Source: three-view drawing plus pictorial views. Frame: mm from the lowest corner of the part. A direction names the side the tool comes from. Give positions to 0.01 mm unless a question says otherwise; leave off trailing zeros. Order: outer loops, then holes, each group sorted by start corner. A loop starts at its lowest first (then second) coordinate and runs counter-clockwise, first axis right, second up. Notation, with made-up numbers: M 46,5 L 81,5 A18 cw 81,19 Z; hole C 11,76 d5. An arc over 180 degrees is marked long. Use CSV: the item, a comma, the result in double quotes. Start each with the question number.
1. Pin query (flat end, axial travel): P1, Ø5, axis at y = 7, z = 62, coming from the -X side (1 decimal); P2, Ø4, axis at x = 26.5, z = 35.5, coming from the -Y side; P3, Ø2.5, axis at x = 35, z = 20, coming from the +Y side; P4, Ø8, axis at x = 27.5, z = 44, coming from the +Y side. Return the tip coordinate at first contact, or that it passes through.
2. Mould query, pull axis Z, two halves, no side actions, for the marked faces 4, 5, 6 and 7. Classes: released by +Z, released by -Z, zero draft, split by the parting line, or undercut.
3. Section query D-D, the plane z = 50. Return the cut outline in (x, y).
4. Reachability of the marked faces 1, 2 and 3 from +Z, -Z, +X, -X, +Y, -Y: full face, straight path, thin tool, end or side. Return the list, or none.
5. Line query: line 1 along Z through (x, y) = (14.5, 9.5); line 2 along Y through (x, z) = (46.5, 21.5); line 3 along Z through (x, y) = (23.5, 7.75) (1 decimal). Output: solid intervals per line, ascending. Write a range as [from, to].
6. Section query A-A, the plane x = 35. Return the cut outline in (y, z).
7. Section query B-B, the plane y = 7. State how many separate pieces and enclosed holes the cut face has, plus the area to 3 significant figures.
8. Section query C-C, the plane z = 36. Return the cut outline in (x, y) (1 decimal), plus the area to 3 significant figures.
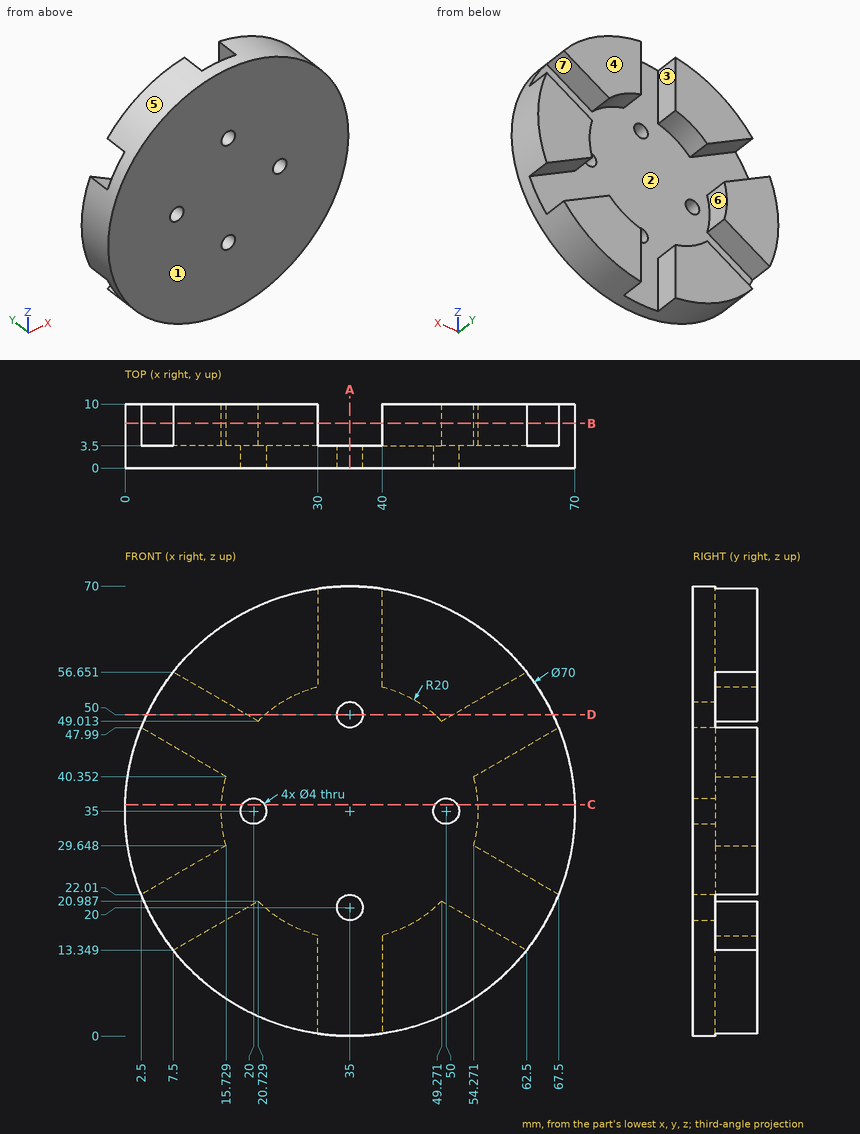
Result set:
1,P1,"x = 10"
1,P2,"y = 0"
1,P3,"through"
1,P4,"y = 3.5"
2,face 4,"zero draft"
2,face 5,"split by the parting line"
2,face 6,"undercut"
2,face 7,"undercut"
3,outline,"M 3.38,0 L 33,0 L 33,3.5 L 21.77,3.5 L 21.77,10 L 19.02,10 L 19.02,3.5 L 3.38,3.5 Z; M 37,0 L 66.62,0 L 66.62,3.5 L 50.98,3.5 L 50.98,10 L 48.23,10 L 48.23,3.5 L 37,3.5 Z"
4,face 1,"+Z, -Z, +X, -X, -Y"
4,face 2,"+Y"
4,face 3,"+Z, -Z, +Y"
5,line 1,"[6.63, 17.39], [28.94, 41.06], [52.61, 63.37]"
5,line 2,"[0, 3.5]"
5,line 3,"[1.9, 18.6], [51.4, 68.1]"
6,outline,"M 0,0 L 3.5,0 L 3.5,18 L 0,18 Z; M 0,22 L 3.5,22 L 3.5,48 L 0,48 Z; M 0,52 L 3.5,52 L 3.5,70 L 0,70 Z"
7,separate pieces,"6"
7,enclosed holes,"0"
7,area,"1,690 mm2"
8,outline,"M 0,0 L 18.3,0 L 18.3,3.5 L 15,3.5 L 15,10 L 0,10 Z; M 21.7,0 L 48.3,0 L 48.3,3.5 L 21.7,3.5 Z; M 51.7,0 L 70,0 L 70,10 L 55,10 L 55,3.5 L 51.7,3.5 Z"
8,area,"416 mm2"
